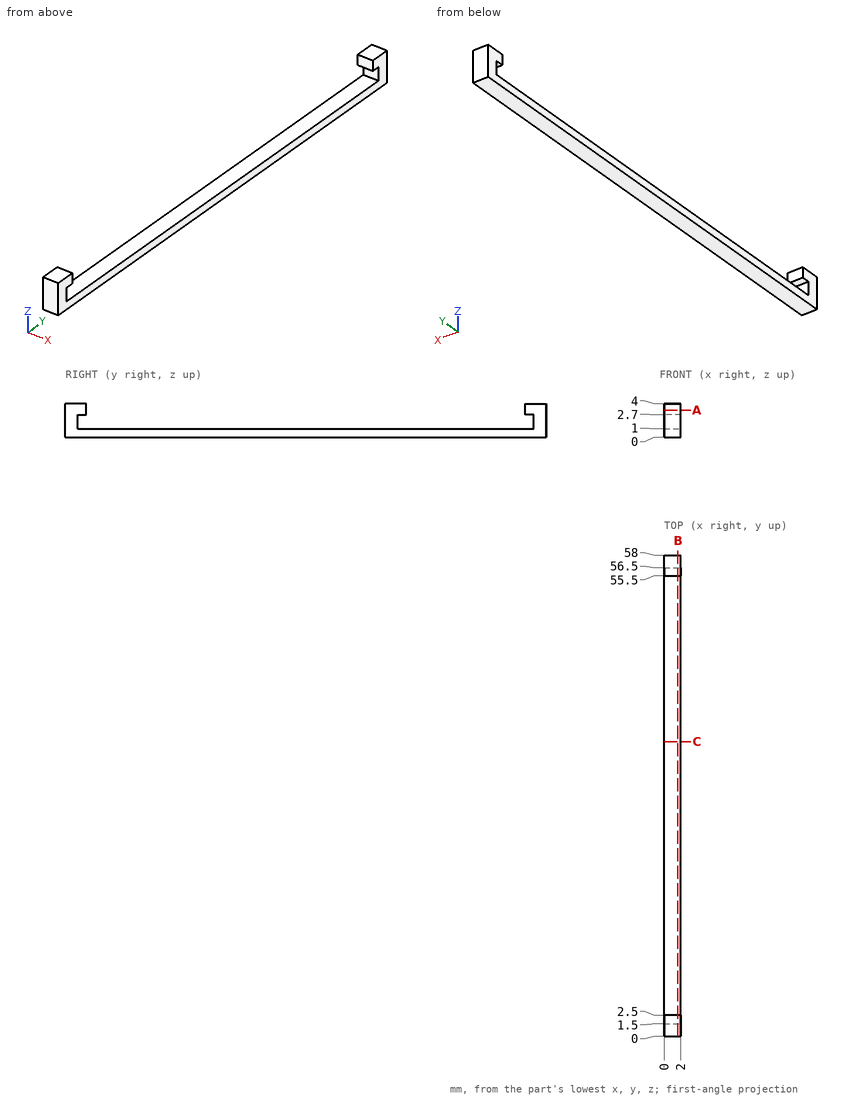
Job drawing, mm, ordinate dimensions from the low corner. One solid piece. Give positions to 0.01 mm unless a question says otherwise; leave off trailing zeros. Write each loop counter-clockwise with the first axis right and the second up, starting at its lowest first coordinate (ties: lowest second). Pieces come first, ordered by that corner, then holes. Notation, with made-up numbers: (-9, -8) - (-2, -8) arc R18 ccw to (-2, 16) - close; hole circle Ø4 at (-39, -26). An arc over 180 degrees is marked (long way). Use one line per item in the form item = value. Start each with the question number.
1. Band-saw the part on C-C on y = 35.5. Write the cut outline in (x, z), plus the area to 3 significant figures.
2. Band-saw the part on A-A on z = 3.25. Write the cut outline in (x, y), plus the area to 3 significant figures.
3. Probe line 1 (Y direction, x = 1, z = 1.3); line 2 (Y direction, x = 1.6, z = 3.2); line 3 (Z direction, x = 1.6, y = 15.5). List the from-to ranges inside material, lowest first. Write a range as [from, to].
4. Drop a flat-ended pin along its axis: pin 1 Ø1 at (x, y) = (0.5, 37.5) entering from +Z. Give the stop position or say it passes through.
5. Band-saw the part on B-B on x = 1.65. Write the cut outline in (y, z).
Conclusion:
q1.outline = (0, 0) - (2, 0) - (2, 1) - (0, 1) - close
q1.area = 2.00 mm²
q2.outline = (0, 0) - (2, 0) - (2, 2.5) - (0, 2.5) - close; (0, 55.5) - (2, 55.5) - (2, 58) - (0, 58) - close
q2.area = 10.0 mm²
q3.line_1 = [0, 1.5], [56.5, 58]
q3.line_2 = [0, 2.5], [55.5, 58]
q3.line_3 = [0, 1]
q4.pin_1 = 1
q5.outline = (0, 0) - (58, 0) - (58, 4) - (55.5, 4) - (55.5, 2.7) - (56.5, 2.7) - (56.5, 1) - (1.5, 1) - (1.5, 2.7) - (2.5, 2.7) - (2.5, 4) - (0, 4) - close
